Geometry: final body of the model. Coordinates: model frame, mm. Face numbers are marked on the shaded views. A direction names the side the tool comes from. Round coordinates to 2 decimals unless told otherwise and drop trailing zeros. Loops run counter-clockwise (first coordinate to the right, second up) from the corner with the lowest first, then second, coordinate; pieces in that order, holes last. Notation, with made-up numbers: (52, 74) - (56, 74) arc R17 ccw to (56, 91) - close; hole circle Ø5 at (-6, 13). An arc over 180 degrees is marked (long way). Answer as a JSON object with one key per item and string values. Group by question number.
Item 1: Section D-D (y = 114). Return the cut outline in (x, z).
Item 2: Section B-B (x = 0). Return the cut outline in (y, z).
Item 3: Section C-C (z = 216). Return the cut outline in (x, y).
Item 4: First-contact query: pin 1 (3 mm diameter, centred on x = -121.5, z = 104, fed in from +Y); pin 2 (8 mm diameter, centred on x = -93, z = 361.5, fed in from -Y); pin 3 (6 mm diameter, centred on y = -101, z = 360.5, fed in from +X). Flat tips, straight axial feed; report the tip coordinate or a pass-through.
Item 5: Reachability of the marked faces 1 and 2 from +Z, -Z, +X, -X, +Y, -Y: full face, straight path, thin tool, end or side. Return the list, or none.
Item 6: Section A-A (y = 0). Return the cut outline in (x, z).
Item 7: Draft query along Z for the marked faces 3, 4, 5 and 6. Return one class per face: released by +Z, released by -Z, zero draft, split by the parting line, or undercut.
Item 8: Line query: line 1 (Y direction, x = 0, z = 1.5); line 2 (Z direction, x = 69, y = -17.5); line 3 (X direction, y = 82, z = 423). Output: solid intervals per line, ascending.
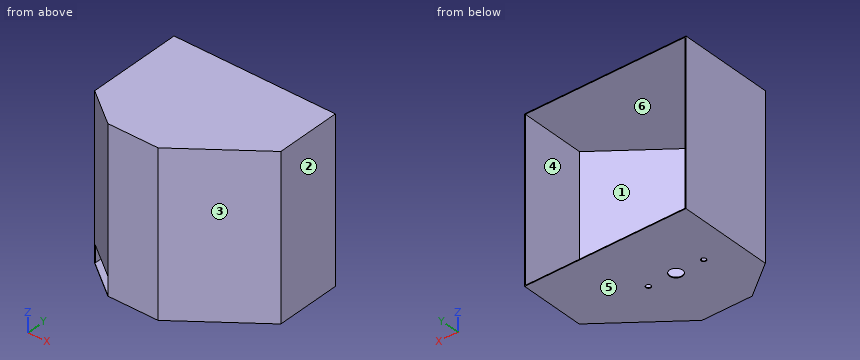
```python
from build123d import *

# Parameters (mm, degrees)
SALIENTE_EXTRUIR1_DEPTH = 2
SALIENTE_EXTRUIR2_DEPTH = 450
SALIENTE_EXTRUIR3_DEPTH = 2
CROQUIS4_R              = 18
CORTAR_EXTRUIR1_DEPTH   = 2
CROQUIS5_W              = 123.547211961
CROQUIS5_H              = 50
CORTAR_EXTRUIR2_DEPTH   = 2
CROQUIS6_R              = 7
CORTAR_EXTRUIR3_DEPTH   = 2


with BuildPart() as part:
    # Croquis1 → Saliente-Extruir1 (new body)
    with BuildSketch(Plane.XY):
        Polygon((-70, -170), (70, -170), (280, -11.753649478), (280, 170), (-170, 170), (-170, -94.64459499), align=None)
    extrude(amount=SALIENTE_EXTRUIR1_DEPTH)

    # Croquis2 → Saliente-Extruir2 (add)
    with BuildSketch(Plane.XY.offset(2)):
        Polygon((-170, 170), (-168, 170), (-168, -93.647431774), (-69.330809361, -168), (69.330809361, -168), (278, -10.756486262), (278, 170), (280, 170), (280, -11.753649478), (70, -170), (-70, -170), (-170, -94.64459499), align=None)
    extrude(amount=SALIENTE_EXTRUIR2_DEPTH)

    # Croquis3 → Saliente-Extruir3 (add)
    with BuildSketch(Plane.XY.offset(452)):
        Polygon((-170, 170), (280, 170), (280, -11.753649478), (70, -170), (-70, -170), (-170, -94.64459499), align=None)
    extrude(amount=-SALIENTE_EXTRUIR3_DEPTH)

    # Croquis4 → Cortar-Extruir1 (cut)
    with BuildSketch(Plane.XY.offset(2)):
        Circle(CROQUIS4_R)
    extrude(amount=-CORTAR_EXTRUIR1_DEPTH, mode=Mode.SUBTRACT)

    # Croquis5 → Cortar-Extruir2 (cut)
    with BuildSketch(Plane(origin=(-105.856306655, -140.476063582, 0), x_dir=(0.7986355100472919, -0.6018150231520497, 0), z_dir=(0.6018150231520497, 0.7986355100472919, 0))):
        with Locations((-16.038728387, -27)):
            Rectangle(CROQUIS5_W, CROQUIS5_H)
    extrude(amount=-CORTAR_EXTRUIR2_DEPTH, mode=Mode.SUBTRACT)

    # Croquis6 → Cortar-Extruir3 (cut)
    with BuildSketch(Plane(origin=(0, 0, 0), x_dir=(-1, 0, 0), z_dir=(0, 0, -1))):
        with Locations((77, 0)):
            Circle(CROQUIS6_R)
        with Locations(Location((-77, 0, 0), (0, 0, 180))):
            Circle(CROQUIS6_R)
    extrude(amount=-CORTAR_EXTRUIR3_DEPTH, mode=Mode.SUBTRACT)


solid = part.part
```
Values:
{
 "1": {"outline": "(-170, 0) - (280, 0) - (280, 452) - (-170, 452) - close; hole (-168, 2) - (278, 2) - (278, 450) - (-168, 450) - close"},
 "2": {"outline": "(-170, 0) - (-18, 0) - (-18, 2) - (-168, 2) - (-168, 450) - (170, 450) - (170, 452) - (-170, 452) - close; (18, 0) - (170, 0) - (170, 2) - (18, 2) - close"},
 "3": {"outline": "(-170, -94.64) - (-70, -170) - (70, -170) - (280, -11.75) - (280, 170) - (278, 170) - (278, -10.76) - (69.33, -168) - (-69.33, -168) - (-168, -93.65) - (-168, 170) - (-170, 170) - close"},
 "4": {"pin 1": "stops at y = -127.56", "pin 2": "stops at y = -155.68", "pin 3": "stops at x = 165.55"},
 "5": {"face 1": "+Y", "face 2": "+Z, -Z, +X, +Y, -Y"},
 "6": {"outline": "(-170, 0) - (-84, 0) - (-84, 2) - (-168, 2) - (-168, 450) - (278, 450) - (278, 2) - (84, 2) - (84, 0) - (280, 0) - (280, 452) - (-170, 452) - close; (-70, 0) - (-18, 0) - (-18, 2) - (-70, 2) - close; (18, 0) - (70, 0) - (70, 2) - (18, 2) - close"},
 "7": {"face 3": "zero draft", "face 4": "undercut", "face 5": "released by -Z", "face 6": "undercut"},
 "8": {"line 1": "y = -170 to -18, 18 to 170", "line 2": "z = 0 to 2, 450 to 452", "line 3": "x = -170 to -168, 278 to 280"}
}
